Source: CAD feature listing. Evaluate the final solid. Frame: model axes, mm. Face numbers are marked on the shaded views. A direction names the side the tool comes from. Give positions to 0.01 mm unless a question says otherwise; leave off trailing zeros. Loops run counter-clockwise (first coordinate to the right, second up) from the corner with the lowest first, then second, coordinate; pieces in that order, holes last. Notation, with made-up numbers: (30, -10) -> (34, -10) arc R17 cw to (34, 23) -> close; hole circle Ø7 at (-37, 35.25). An arc over 180 degrees is marked (long way). Put each result on its own line as item: value.
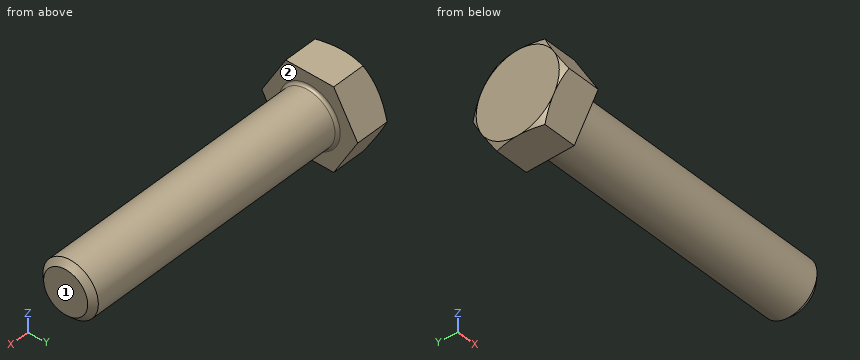
Autodesk Inventor part; units mm, degrees
ref_plane "Work Plane1" through (1.525, 0, 0) normal (0, 0, 1) x (1, 0, 0)
ref_plane "YZ Plane" through (0, 0, 0) normal (1, 0, 0) x (0, 1, 0)
ref_plane "XZ Plane" through (0, 0, 0) normal (0, 1, 0) x (-1, 0, 0)
sketch "Sketch1" plane through (0, 0, 0) normal (0, 0, 1) x (1, 0, 0)
  line L0 (0, 3) -> (30, 3)
  line L1 (30, 3) -> (30, 0)
  line L2 (30, 0) -> (0, 0)
  line L3 (-6, 0) -> (36, 0)
  line L4 (0, -0.6) -> (0, 3.6)
  line L5 (0, 3) -> (0, 0)
  dimension "d2" = 6
  dimension "d59" = 30
revolve "Body" add sketch "Sketch1" angle 360 about axis through (30, 0, 0) along (-1, 0, 0)
sketch "Sketch2" plane through (0, 0, 0) normal (-1, 0, 0) x (0, 0, 1)
  line L0 (0, 5.1962) -> (4.5, 2.5981)
  line L1 (4.5, 2.5981) -> (4.5, -2.5981)
  line L2 (4.5, -2.5981) -> (0, -5.1962)
  line L3 (0, -5.1962) -> (-4.5, -2.5981)
  line L4 (-4.5, -2.5981) -> (-4.5, 2.5981)
  line L5 (-4.5, 2.5981) -> (0, 5.1962)
  line L6 (-6.3, 0) -> (6.3, 0)
  line L7 (0, 7.2746) -> (0, -7.2746)
  point P0 (0, 0)
  point P1 (0, 0)
  dimension "d11" = 9
extrude "Head" add sketch "Sketch2" along normal blind 4
sketch "Sketch4" plane through (0, 0, 0) normal (0, 0, 1) x (1, 0, 0)
  line L0 (-3.4804, 5.4) -> (-4, 4.5)
  line L1 (-1.1, 0) -> (-0.234, 0)
  line L2 (-4.7532, 0) -> (0.5192, 0)
  line L3 (-4, 5.4) -> (-3.4804, 5.4)
  line L4 (-4, 4.5) -> (-4, 5.4)
  line L5 (0, 6.48) -> (0, -1.08)
  dimension "d65" = 9
  dimension "d67" = 30
  dimension "d68" = 10.8
  dimension "d69" = 4
revolve "Chamfer1" cut sketch "Sketch4" angle 360 about axis through (-1.1, 0, 0) along (1, 0, 0)
thread "Thread"
chamfer "Chamfer2" distance 0.6135 distance2 0.6136 1 edges at (30, -3, 0) measured on face at (30, -0.5525, 1.8157)
fillet "Fillet2" radius 0.3 1 edges at (0, -3, 0)
ref_plane "Work Plane1" through (1.525, 0, 0) normal (0, 0, 1) x (1, 0, 0)
equation "\"d71\" = RR"
equation "\"d11\" = SW"
equation "\"d3\" = KOH"
equation "\"d15\" = GEL"
equation "\"d6\" = -0.5 * SPD + 0.5 * GD"
equation "\"d2\" = GD"
equation "\"d59\" = NLG"
equation "\"d65\" = SW"
equation "\"d67\" = ANG1"
equation "\"d68\" = 1.2 * SW"
equation "\"d69\" = KOH"
equation "\"NLG\" = 30"
equation "\"GD\" = NND"
equation "\"BDM\" = NND"
equation "\"KOH\" = 4"
equation "\"GEL\" = 11"
equation "\"SW\" = 9"
equation "\"SW0\" = 9"
equation "\"SPD\" = NND - 1.2269 * PTC"
equation "\"SD2\" = NND"
equation "\"SD\" = 0"
equation "\"ANG1\" = 30deg"
equation "\"GAL\" = 0.61345 * PTC"
equation "\"GUL\" = 0.61345 * PTC"
equation "\"RR\" = 0.3"
equation "\"RR1\" = 0.1"
equation "\"GD1\" = THREADDIA - 1.2269 * PTC"
equation "\"THREADDIA\" = 6"
equation "\"TOA\" = 30deg"
equation "\"FAWI\" = 60deg"
equation "\"PTC\" = 1"
equation "\"NND\" = 6"
equation "\"E0\" = 1.155 * SW"
properties part number "CSN 02 1201 - M6 x 30" material "Steel, Mild"
(1) Section A-A on x = 16. Return loops of the section in (y, z), then the cut area to 3 significant figures.
Calculated:
outline: circle Ø6 at (0, 0)
area: 28.3 mm²
(2) First-contact query: P1, Ø2, axis at x = 24, z = 3.5, coming from the -Y side; P2, Ø1, axis at x = 0, z = 1, coming from the +Y side; P3, Ø2, axis at x = 20, y = -2.5, coming from the +Z side. Flat tips, straight axial feed; report the tip coordinate or a pass-through.
Calculated:
P1: stops at y = -1.66
P2: stops at y = 4.91
P3: stops at z = 2.6
(3) Reachability of the marked faces 1 and 2 from +Z, -Z, +X, -X, +Y, -Y: full face, straight path, thin tool, end or side. Return the list, or none.
Calculated:
face 1: +Z, -Z, +X, +Y, -Y
face 2: +X
(4) Line query: probe 1 along Y at (x, z) = (15, 0); probe 2 along X at (y, z) = (0.75, 4.25); probe 3 along Z at (x, y) = (8, -1.5). Output: solid intervals per line, ascending. Write a range as from..to.
Calculated:
probe 1: y = -3..3
probe 2: x = -4..0
probe 3: z = -2.6..2.6
